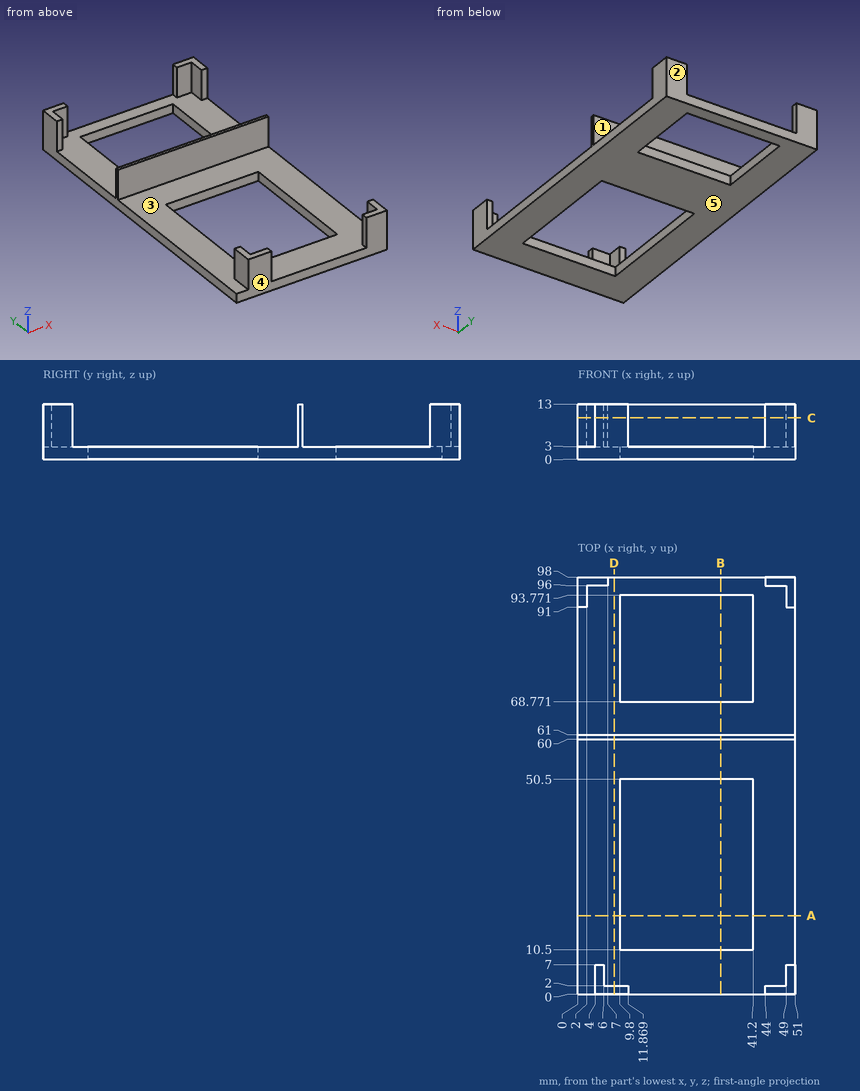
Geometry check sheet. Reference: drawing and pictorial views, mm from the part's lowest x, y, z. A direction names the side the tool comes from. Give positions to 0.01 mm unless a question says otherwise; leave off trailing zeros. Write each loop counter-clockwise with the first axis right and the second up, starting at its lowest first coordinate (ties: lowest second). Pieces come first, ordered by that corner, then holes. Notation, with made-up numbers: (-22.75, 37) -> (-2.75, 37) arc R31 cw to (-2.75, 67) -> close; hole circle Ø6 at (-23.5, 10.25). An arc over 180 degrees is marked (long way). One line per item, written item: value. Start each with the question number.
Item 1: Tool access check on the marked faces 1 and 2. Record the directions out of +Z, -Z, +X, -X, +Y, -Y that give a thin tool (end or side, any length) a straight path to the whole face; none if there is none.
Item 2: Section check D-D on x = 8.5. Record the cut outline in (y, z).
Item 3: Section check A-A on y = 18.5. Record the cut outline in (x, z).
Item 4: Section check C-C on z = 9.75. Record the cut outline in (x, y), then the cut area to 3 significant figures.
Item 5: Gauge pin test, flat ends, axial feed: pin 1 (4 mm diameter, centred on x = 37, z = 11, fed in from +Y); pin 2 (0.6 mm diameter, centred on y = 0.5, z = 6.5, fed in from -X); pin 3 (1 mm diameter, centred on x = 1.5, z = 9, fed in from -Y). Record the tip position at first contact, or that the pin passes through.
Item 6: Material ranges on probe 1 along Y at (x, z) = (48.5, 9.75); probe 2 along Y at (x, z) = (8, 9.75); probe 3 along Y at (x, z) = (39, 7), recorded low to high. Write a range as from..to.
Item 7: Section check B-B on x = 33.5. Record the cut outline in (y, z).
Item 8: Draft check along Y on the marked faces 3, 4 and 5. Enter one of: +Y half, -Y half, draft (parallel to the pull), parting line (faces both ways), or undercut.
Results list:
1. face 1: +Z, +X, -X
1. face 2: +Z, -Z, +X, -X, +Y
2. outline: (0, 0) -> (98, 0) -> (98, 3) -> (61, 3) -> (61, 13) -> (60, 13) -> (60, 3) -> (2, 3) -> (2, 13) -> (0, 13) -> close
3. outline: (0, 0) -> (9.8, 0) -> (9.8, 3) -> (0, 3) -> close; (41.2, 0) -> (51, 0) -> (51, 3) -> (41.2, 3) -> close
4. outline: (0, 60) -> (51, 60) -> (51, 61) -> (0, 61) -> close; (0, 91) -> (2, 91) -> (2, 96) -> (7, 96) -> (7, 98) -> (0, 98) -> close; (4, 0) -> (11.87, 0) -> (11.87, 2) -> (6, 2) -> (6, 7) -> (4, 7) -> close; (44, 0) -> (51, 0) -> (51, 7) -> (49, 7) -> (49, 2) -> (44, 2) -> close; (44, 96) -> (49, 96) -> (49, 91) -> (51, 91) -> (51, 98) -> (44, 98) -> close
4. area: 149 mm²
5. pin 1: y = 61
5. pin 2: x = 4
5. pin 3: y = 60
6. probe 1: 0..2, 60..61, 96..98
6. probe 2: 0..2, 60..61
6. probe 3: 60..61
7. outline: (0, 0) -> (10.5, 0) -> (10.5, 3) -> (0, 3) -> close; (50.5, 0) -> (68.77, 0) -> (68.77, 3) -> (61, 3) -> (61, 13) -> (60, 13) -> (60, 3) -> (50.5, 3) -> close; (93.77, 0) -> (98, 0) -> (98, 3) -> (93.77, 3) -> close
8. face 3: undercut
8. face 4: -Y half
8. face 5: draft
